```python
from build123d import *

# Parameters (mm, degrees)
F0_W     = 19
F0_H     = 42
F0_R     = 1.65
F1_DEPTH = 20
F3_DEPTH = 3
F2_R     = 2.1
F4_DEPTH = 22
F2_R_2   = 3.6
F5_DEPTH = 15
F6_R     = 3


with BuildPart() as f1:
    # F0 (on Top) → F1 (new body)
    with BuildSketch(Plane.XY):
        Rectangle(F0_W, F0_H)
        with Locations((-5, -13)):
            Circle(F0_R, mode=Mode.SUBTRACT)
        with Locations((5, -13)):
            Circle(F0_R, mode=Mode.SUBTRACT)
        with Locations((-5, 13)):
            Circle(F0_R, mode=Mode.SUBTRACT)
        with Locations((5, 13)):
            Circle(F0_R, mode=Mode.SUBTRACT)
    extrude(amount=F1_DEPTH)

    # F3 (add): a face of the model
    f3_faces = [f1.faces().sort_by_distance(p)[0] for p in [
        (-9.5, 0, 10),
    ]]
    extrude(f3_faces, amount=F3_DEPTH)

    # F2 (on face) → F4 (cut, through all)
    with BuildSketch(Plane.YZ.offset(9.5)):
        with Locations((-6.415, 15.07)):
            Circle(F2_R)
        with Locations((6.415, 15.07)):
            Circle(F2_R)
        with Locations((6.415, 4.93)):
            Circle(F2_R)
        with Locations((-6.415, 4.93)):
            Circle(F2_R)
    extrude(amount=-F4_DEPTH, mode=Mode.SUBTRACT)

    # F2 (on face) → F5 (cut)
    with BuildSketch(Plane.YZ.offset(9.5)):
        with Locations((6.415, 15.07)):
            Circle(F2_R_2)
        with Locations((6.415, 15.07)):
            Circle(F2_R, mode=Mode.SUBTRACT)
        with Locations((6.415, 4.93)):
            Circle(F2_R_2)
        with Locations((6.415, 4.93)):
            Circle(F2_R, mode=Mode.SUBTRACT)
        with Locations((-6.415, 4.93)):
            Circle(F2_R_2)
        with Locations((-6.415, 4.93)):
            Circle(F2_R, mode=Mode.SUBTRACT)
        with Locations((-6.415, 15.07)):
            Circle(F2_R_2)
        with Locations((-6.415, 15.07)):
            Circle(F2_R, mode=Mode.SUBTRACT)
    extrude(amount=-F5_DEPTH, mode=Mode.SUBTRACT)

    # F6
    f6_edges = [f1.edges().sort_by_distance(p)[0] for p in [
        (-1.5, 21, 0),
        (-1.5, -21, 0),
        (-1.5, -21, 20),
        (-1.5, 21, 20),
    ]]
    fillet(f6_edges, radius=F6_R)


solid = f1.part
```
Read the model definition and answer for the solid it produces. Units are mm, in the model's axes. A direction names the side the tool comes from. Coordinates: 2 decimals unless noted, no trailing zeros. Order: outer loops, then holes, each group sorted by start corner. A loop starts at its lowest first (then second) coordinate and runs counter-clockwise, first axis right, second up. Notation, with made-up numbers: (49.5, 84.25) - (66.5, 84.25) arc R13 cw to (66.5, 93.25) - close; hole circle Ø9 at (86.25, 15). An arc over 180 degrees is marked (long way). Answer as a JSON object with one key per item and string values. Group by question number.
Item 1: Section D-D (x = -1.5) is taken. Give the vertices of the cut face in (y, z) (3 decimals).
Item 2: Flat-ended cylindrical pins translate along their axes: P1, Ø6.5, axis at y = 6.415, z = 4.93, coming from the +X side; P2, Ø2.5, axis at y = -6.415, z = 15.07, coming from the +X side; P3, Ø1, axis at x = 6.5, z = 18, coming from the -Y side. Find the tip coordinate at first contact, or state that the pin passes through.
Item 3: Section B-B (z = 4.93) is taken. Give the vertices of the cut face in (x, y) (3 decimals), plus the area to 3 significant figures.
Item 4: Consider probe 1 along Y at (x, z) = (6.25, 18); probe 2 along Y at (x, z) = (7, 5.25); probe 3 along Y at (x, z) = (-5, 13.75). Determine where each line is inside the solid, lowest interval first. Write a range as from..to.
Item 5: The mould has two halves that part along Y. Classify faces 3 (the face through (-12.5, 0, 10)), 4 (the face through (-1, 21, 10)), 5 (the face through (2.11, 5.95, 8.5)), 6 (the face through (3.69, -14, 9.86)): +Y half, -Y half, draft (parallel to the pull), parting line (faces both ways), or undercut.
Item 6: Section A-A (x = -5) is taken. Give the vertices of the cut face in (y, z) (3 decimals), plus the area to 3 significant figures.
Item 7: A tool of negligible diameter and unlimited length cuts with its end or side. For faces 1 (the face through (-1.65, -20.14, 19.1)), 2 (the face through (-5.5, -6.5, 12.7)), from which of +Z, -Z, +X, -X, +Y, -Y can it reach the whole face along a straight path? Write none if from no direction.
Item 8: Section C-C (y = 13) is taken. Give the vertices of the cut face in (x, z), plus the area to 3 significant figures.
Results are:
{
 "1": {"outline": "(-21, 3) arc R3 ccw to (-18, 0) - (18, 0) arc R3 ccw to (21, 3) - (21, 17) arc R3 ccw to (18, 20) - (-18, 20) arc R3 ccw to (-21, 17) - close; hole circle Ø7.2 at (-6.415, 4.93); hole circle Ø7.2 at (-6.415, 15.07); hole circle Ø7.2 at (6.415, 4.93); hole circle Ø7.2 at (6.415, 15.07)"},
 "2": {"P1": "stops at x = -5.5", "P2": "passes through", "P3": "stops at y = -20.96"},
 "3": {"outline": "(-12.5, -21) - (9.5, -21) - (9.5, -10.015) - (-5.5, -10.015) - (-5.5, -8.515) - (-12.5, -8.515) - close; (-12.5, -4.315) - (-5.5, -4.315) - (-5.5, -2.815) - (9.5, -2.815) - (9.5, 2.815) - (-5.5, 2.815) - (-5.5, 4.315) - (-12.5, 4.315) - close; (-12.5, 8.515) - (-5.5, 8.515) - (-5.5, 10.015) - (9.5, 10.015) - (9.5, 21) - (-12.5, 21) - close; hole circle Ø3.3 at (-5, -13); hole circle Ø3.3 at (-5, 13); hole circle Ø3.3 at (5, -13); hole circle Ø3.3 at (5, 13)", "area": "615 mm^2"},
 "4": {"probe 1": "y = -20.83..-14.08, -11.92..-8.51, -4.32..4.32, 8.51..11.92, 14.08..20.83", "probe 2": "y = -21..-10, -2.83..2.83, 10..21", "probe 3": "y = -21..-14.65, -11.35..-9.76, -3.07..3.07, 9.76..11.35, 14.65..21"},
 "5": {"face 3": "draft", "face 4": "+Y half", "face 5": "undercut", "face 6": "undercut"},
 "6": {"outline": "(-21, 3) arc R3 ccw to (-18, 0) - (-14.65, 0) - (-14.65, 20) - (-18, 20) arc R3 ccw to (-21, 17) - close; (-11.35, 0) - (11.35, 0) - (11.35, 20) - (-11.35, 20) - close; (14.65, 0) - (18, 0) arc R3 ccw to (21, 3) - (21, 17) arc R3 ccw to (18, 20) - (14.65, 20) - close; hole circle Ø7.2 at (-6.415, 4.93); hole circle Ø7.2 at (-6.415, 15.07); hole circle Ø7.2 at (6.415, 4.93); hole circle Ø7.2 at (6.415, 15.07)", "area": "537 mm^2"},
 "7": {"face 1": "+Z, +X, -X, -Y", "face 2": "+X"},
 "8": {"outline": "(-12.5, 0) - (-6.65, 0) - (-6.65, 20) - (-12.5, 20) - close; (-3.35, 0) - (3.35, 0) - (3.35, 20) - (-3.35, 20) - close; (6.65, 0) - (9.5, 0) - (9.5, 20) - (6.65, 20) - close", "area": "308 mm^2"}
}
